Model file for the job. Use its own axes, mm. A direction names the side the tool comes from. Coordinates: 2 decimals unless noted, no trailing zeros. Order: outer loops, then holes, each group sorted by start corner. A loop starts at its lowest first (then second) coordinate and runs counter-clockwise, first axis right, second up.
from build123d import *

# Parameters (mm, degrees)
EXTRUDE_2_DEPTH     = 13.5
SKETCH_3_R          = 6
CUT_EXTRUDE_1_DEPTH = 162.383859168
CUT_EXTRUDE_START   = 9
SKETCH_3_3_R        = 8
CUT_EXTRUDE_2_DEPTH = 153.383859168
SKETCH_3_4_R        = 13.5
CUT_EXTRUDE_3_DEPTH = 7.5
FILLET_1_R          = 4
SKETCH_3_5_R        = 21
CUT_EXTRUDE_5_DEPTH = 10.5
SKETCH_3_6_R        = 23.5
CUT_EXTRUDE_7_DEPTH = 7


with BuildPart() as part:
    # Эскиз2 → Бобышка-Вытянуть2 (new body)
    with BuildSketch(Plane.XY):
        with BuildLine():
            ThreePointArc((-31.381638839, 116.547619048), (-25.062561701, 85.800741423), (-22.494803062, 54.516434893))
            ThreePointArc((-22.494803062, 54.516434893), (0, 32.5), (22.494803062, 54.516434893))
            ThreePointArc((22.494803062, 54.516434893), (25.062561701, 85.800741423), (31.381638839, 116.547619048))
            ThreePointArc((31.381638839, 116.547619048), (0, 157.5), (-31.381638839, 116.547619048))
        make_face()
    extrude(amount=EXTRUDE_2_DEPTH)

    # Эскиз3 → Вырез-Вытянуть1 (cut, through all)
    with BuildSketch(Plane.XY):
        with Locations((0, 55)):
            Circle(SKETCH_3_R)
    extrude(amount=CUT_EXTRUDE_1_DEPTH, mode=Mode.SUBTRACT)

    # Эскиз3<3> → Вырез-Вытянуть2 (cut, through all)
    with BuildSketch(Plane.XY.offset(CUT_EXTRUDE_START)):
        with Locations((0, 55)):
            Circle(SKETCH_3_3_R)
    extrude(amount=CUT_EXTRUDE_2_DEPTH, mode=Mode.SUBTRACT)

    # Эскиз3<4> → Вырез-Вытянуть3 (cut)
    with BuildSketch(Plane.XY):
        with Locations((0, 55)):
            Circle(SKETCH_3_4_R)
    extrude(amount=CUT_EXTRUDE_3_DEPTH, mode=Mode.SUBTRACT)

    # Скругление1
    fillet_1_edges = [part.edges().sort_by_distance(p)[0] for p in [
        (25.062561701, 85.800741423, 13.5),
        (0, 157.5, 13.5),
        (-25.062561701, 85.800741423, 13.5),
        (0, 32.5, 13.5),
    ]]
    fillet(fillet_1_edges, radius=FILLET_1_R)

    # Эскиз3<5> → Вырез-Вытянуть5 (cut)
    with BuildSketch(Plane.XY):
        with Locations(Location((0, 125, 0), (0, 0, 180))):
            Circle(SKETCH_3_5_R)
    extrude(amount=CUT_EXTRUDE_5_DEPTH, mode=Mode.SUBTRACT)

    # Эскиз3<6> → Вырез-Вытянуть7 (cut)
    with BuildSketch(Plane.XY):
        with Locations((0, 125)):
            Circle(SKETCH_3_6_R)
    extrude(amount=CUT_EXTRUDE_7_DEPTH, mode=Mode.SUBTRACT)


solid = part.part
Q1. Which spindle directions (+Z, -Z, +X, -X, +Y, -Y) get a long thin tool onto all of the face, cutting with end or side? Do faces 4 (the face through (7.26, 66.38, 3.7)), 5 (the face through (-2, 61, 9)), 6 (the face through (25, 85.37, 4.68)). Say none if no direction does.
Established:
face 4: -Z
face 5: +Z
face 6: +Z, -Z, +X, -Y
Q2. Probe line 1 (X direction, y = 125, z = 9.3); line 2 (X direction, y = 55, z = 8.3); line 3 (Y direction, x = -18, z = 2.5). List the from-to ranges inside material, lowest first.
Established:
line 1: x = -32.5 to -21, 21 to 32.5
line 2: x = -22.51 to -6, 6 to 22.51
line 3: y = 41.5 to 109.89, 140.11 to 152.06
Q3. Cut at A-A, the plane x = 0. List the corners of the cut face in (y, z), plus the area to 3 significant figures.
Established:
outline: (32.5, 0) - (41.5, 0) - (41.5, 7.5) - (49, 7.5) - (49, 9) - (47, 9) - (47, 13.5) - (36.5, 13.5) arc R4 ccw to (32.5, 9.5) - close; (61, 7.5) - (68.5, 7.5) - (68.5, 0) - (101.5, 0) - (101.5, 7) - (104, 7) - (104, 10.5) - (146, 10.5) - (146, 7) - (148.5, 7) - (148.5, 0) - (157.5, 0) - (157.5, 9.5) arc R4 ccw to (153.5, 13.5) - (63, 13.5) - (63, 9) - (61, 9) - close
area: 912 mm2
Q4. Cut at B-B, the plane z = 5.5. List the corners of the cut face in (x, y).
Established:
outline: (-31.38, 116.55) arc R260 cw to (-22.49, 54.52) arc R22.5 ccw to (22.49, 54.52) arc R260 cw to (31.38, 116.55) arc R32.5 ccw (long way) to start; hole circle Ø47 at (0, 125); hole circle Ø27 at (0, 55)
Q5. Drop flat-ended pins along their axis: P1, Ø8, axis at x = 11, z = 11, coming from the +Y side; P2, Ø4, axis at x = -10, z = 4, coming from the +Y side; P3, Ø6, axis at y = 116.5, z = 7.5, coming from the -X side. Give the stop position or say it passes through.
Established:
P1: stops at y = 156.68
P2: stops at y = 156.5
P3: stops at x = -32.03
Q6. Mould opens along X. For faces 1 (the face through (-20.03, 118.69, 8.73)), 2 (the face through (-25.125, 86.236, 4.684)), 3 (the face through (0.83, 157.49, 4.68)) say: pulls with the +X half, pulls with the -X half, needs draft (parallel to the pull), parting line crosses it, or undercut.
Established:
face 1: undercut
face 2: pulls with the -X half
face 3: parting line crosses it
